For this review, take the finished solid that the model builds, in its own axes (mm). A direction names the side the tool comes from. Round coordinates to 2 decimals unless told otherwise and drop trailing zeros. Write each loop counter-clockwise with the first axis right and the second up, starting at its lowest first coordinate (ties: lowest second). Pieces come first, ordered by that corner, then holes. Notation, with made-up numbers: M -21,-33.5 L 37,-33.5 A9 cw 37,-16.5 Z; hole C 43.25,-12 d6. An arc over 180 degrees is marked long. Answer in a Markdown table with one row per item.
```python
from build123d import *

# Parameters (mm, degrees)
PAD_DEPTH       = 18
FILLET_R        = 5
FILLET001_R     = 5
FILLET002_R     = 1
FILLET003_R     = 1
CHAMFER_SIZE    = 7
CHAMFER001_SIZE = 7
SKETCH001_W     = 15
SKETCH001_H     = 15
POCKET_DEPTH    = 10
SKETCH005_R     = 1
POCKET001_DEPTH = 8
SKETCH006_R     = 1
POCKET002_DEPTH = 8
POCKET003_DEPTH = 18
CHAMFER002_SIZE = 1
CHAMFER003_SIZE = 1


with BuildPart() as part:
    # Sketch → Pad (new body)
    with BuildSketch(Plane(origin=(0, 0, 0), x_dir=(1, 0, 0), z_dir=(0, 0, -1))):
        Polygon((206.173076, -21.002959), (196.173076, -21.002959), (188.480768, -50), (0, 0), (7.692308, 28.997041), (-10, 28.997041), (-10, -69.999032), (206.173076, -69.999032), align=None)
    extrude(amount=PAD_DEPTH)

    # Fillet
    fillet_edges = [part.edges().sort_by_distance(p)[0] for p in [
        (7.692308, -28.997041, -9),
    ]]
    fillet(fillet_edges, radius=FILLET_R)

    # Fillet001
    fillet001_edges = [part.edges().sort_by_distance(p)[0] for p in [
        (196.173076, 21.002959, -9),
    ]]
    fillet(fillet001_edges, radius=FILLET001_R)

    # Fillet002
    fillet002_edges = [part.edges().sort_by_distance(p)[0] for p in [
        (206.173076, 21.002959, -9),
    ]]
    fillet(fillet002_edges, radius=FILLET002_R)

    # Fillet003
    fillet003_edges = [part.edges().sort_by_distance(p)[0] for p in [
        (-10, -28.997041, -9),
    ]]
    fillet(fillet003_edges, radius=FILLET003_R)

    # Chamfer
    chamfer_edges = [part.edges().sort_by_distance(p)[0] for p in [
        (0, 0, -9),
    ]]
    chamfer(chamfer_edges, length=CHAMFER_SIZE)

    # Chamfer001
    chamfer001_edges = [part.edges().sort_by_distance(p)[0] for p in [
        (188.480768, 50, -9),
    ]]
    chamfer(chamfer001_edges, length=CHAMFER001_SIZE)

    # Sketch001 → Pocket (cut)
    with BuildSketch(Plane.XY):
        with Locations((12.5, 47.499032)):
            Rectangle(SKETCH001_W, SKETCH001_H)
        with Locations((97.5, 47.499032)):
            Rectangle(SKETCH001_W, SKETCH001_H)
    extrude(amount=-POCKET_DEPTH, mode=Mode.SUBTRACT)

    # Sketch005 → Pocket001 (cut)
    with BuildSketch(Plane.XY.offset(-10)):
        with Locations((12.5, 47.499032)):
            Circle(SKETCH005_R)
    extrude(amount=-POCKET001_DEPTH, mode=Mode.SUBTRACT)

    # Sketch006 → Pocket002 (cut)
    with BuildSketch(Plane.XY.offset(-10)):
        with Locations((97.5, 47.499032)):
            Circle(SKETCH006_R)
    extrude(amount=-POCKET002_DEPTH, mode=Mode.SUBTRACT)

    # Sketch004 → Pocket003 (cut)
    with BuildSketch(Plane(origin=(0, 0, -18), x_dir=(1, 0, 0), z_dir=(0, 0, -1))):
        Polygon((85.452662, -28.876331), (172.443786, -51.953254), (173.982248, -46.153846), (86.991124, -23.076923), align=None)
    extrude(amount=-POCKET003_DEPTH, mode=Mode.SUBTRACT)

    # Chamfer002
    chamfer002_edges = [part.edges().sort_by_distance(p)[0] for p in [
        (86.991124, 23.076923, -9),
    ]]
    chamfer(chamfer002_edges, length=CHAMFER002_SIZE)

    # Chamfer003
    chamfer003_edges = [part.edges().sort_by_distance(p)[0] for p in [
        (173.982248, 46.153846, -9),
    ]]
    chamfer(chamfer003_edges, length=CHAMFER003_SIZE)


solid = part.part
```
Q1. Take a section at A-A (z = -5.75). State the section outline as (x, y) points.
Found:
| item | result |
|---|---|
| outline | M -10,-28 A1 ccw -9,-29 L 1.19,-29 A5 ccw 6.03,-22.71 L 1.79,-6.77 L 6.77,1.79 L 86.02,22.82 L 86.73,24.04 L 85.45,28.88 L 172.44,51.95 L 173.73,47.12 L 174.95,46.41 L 181.71,48.21 L 190.28,43.23 L 195.19,24.72 A5 ccw 200.02,21 L 205.17,21 A1 ccw 206.17,22 L 206.17,70 L -10,70 Z; hole M 5,40 L 20,40 L 20,55 L 5,55 Z; hole M 90,40 L 105,40 L 105,55 L 90,55 Z |
Q2. Machinability: for faces 4 (the face through (5, 47, -5)), 5 (the face through (3.88, -14.63, -8.87)), 6 (the face through (186.06, 45.68, -8.87)), which of the approach directions +Z, -Z, +X, -X, +Y, -Y give a long, thin tool a straight path to every point of the face, cutting with its end or side? Answer none if there is none.
Found:
| item | result |
|---|---|
| face 4 | +Z |
| face 5 | +Z, -Z, +X |
| face 6 | +Z, -Z, -Y |
Q3. Take a section at B-B (y = -15.5). State the section outline as (x, z) points, then the cut area to 3 significant figures.
Found:
| item | result |
|---|---|
| outline | M -10,-18 L 4.11,-18 L 4.11,0 L -10,0 Z |
| area | 254 mm² |
Q4. For probe 1 along Y at (x, z) = (12.5, -14); probe 2 along Y at (x, z) = (18, -2.5); probe 3 along X at (y, z) = (25.5, -4.25), list the stretches that pass through material, from the lowest coordinate up.
Found:
| item | result |
|---|---|
| probe 1 | 3.32 to 46.5, 48.5 to 70 |
| probe 2 | 4.78 to 40, 55 to 70 |
| probe 3 | -10 to 86.35, 194.98 to 206.17 |
Q5. Insertion check: P1, Ø1.6, axis at x = 12.5, y = 47.5, coming from the +Z side; P2, Ø4, axis at y = -2, z = -3.5, coming from the +X side; P3, Ø1.5, axis at x = 86, z = -2, coming from the -Y side; P4, Ø4.5, axis at x = 98, y = 46.5, coming from the +Z side. Each pin has a flat end and moves straight along its axis. Give the tip position at first contact, or say it passes through.
Found:
| item | result |
|---|---|
| P1 | through |
| P2 | x = 5.72 |
| P3 | y = 22.62 |
| P4 | z = -10 |
Q6. Mouldability with a two-part tool opening along Y and no side actions: class faces 1 (the face through (12, 49, -10)), 2 (the face through (97, 69.999, -9)), 3 (the face through (46.95, 12.455, -8.874)) as +Y half, -Y half, draft (parallel to the pull), parting line (faces both ways), or undercut.
Found:
| item | result |
|---|---|
| face 1 | undercut |
| face 2 | +Y half |
| face 3 | -Y half |
